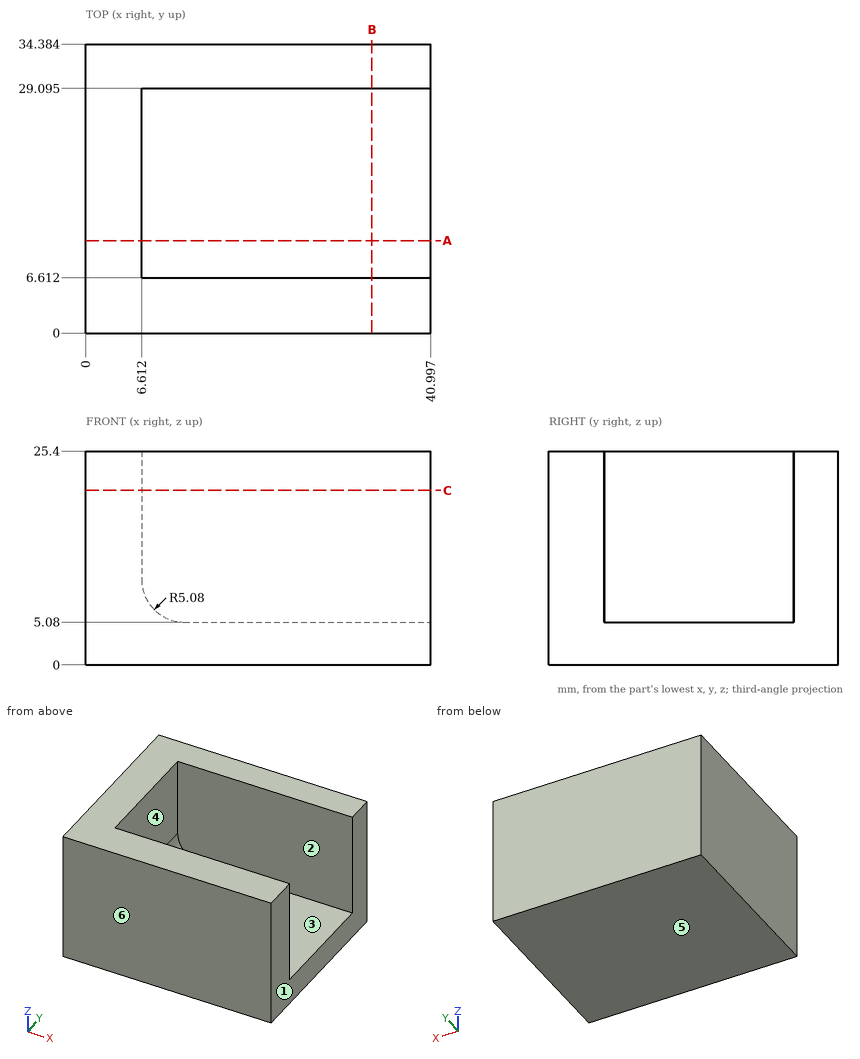
For this review, use the dimensioned drawing (mm, ordinates from the lowest corner) and the shaded views. A direction names the side the tool comes from. Round coordinates to 2 decimals unless told otherwise and drop trailing zeros. Write each loop counter-clockwise with the first axis right and the second up, starting at its lowest first coordinate (ties: lowest second). Pieces come first, ordered by that corner, then holes. Notation, with made-up numbers: M 59.25,44.25 L 75.25,44.25 A10 cw 75.25,49.25 Z; hole C 50,12 d1. An arc over 180 degrees is marked long. Answer as CSV lines item,"result". Start each with the question number.
Q1. Wall thickness on line 1 along Y through (x, z) = (17, 13.75) (1 decimal); line 2 along X through (y, z) = (28, 13.25); line 3 along Z through (x, y) = (36, 7): over which ranges is each line inside the solid? List them lowest first.
Q2. The part is to be moulded in two halves that separate along Y. For the marked faces 3, 4, 5 and 6, say which applies: +Y half, -Y half, draft (parallel to the pull), parting line (faces both ways), or undercut.
Q3. Consider section A-A, the plane y = 11. Give the boundary of the cut face in (x, z), then the cut area to 3 significant figures.
Q4. Clearance check with flat-ended pins moving along their axes: P1, Ø6.5, axis at x = 24, y = 13, coming from the +Z side; P2, Ø4.5, axis at y = 19, z = 15, coming from the +X side. State where each tip first meets the part, or that it passes through.
Q5. Consider section B-B, the plane x = 34. Give the boundary of the cut face in (y, z) (1 decimal).
Q6. Tool access review of the marked faces 1 and 2: name each direction out of +Z, -Z, +X, -X, +Y, -Y from which nothing blocks a thin tool from reaching the whole face with its end or side.
Q7. Consider section C-C, the plane z = 20.75. Give the boundary of the cut face in (x, y) (1 decimal).
Result set:
1,line 1,"y = 0 to 6.6, 29.1 to 34.4"
1,line 2,"x = 0 to 6.61"
1,line 3,"z = 0 to 5.08"
2,face 3,"undercut"
2,face 4,"undercut"
2,face 5,"draft"
2,face 6,"-Y half"
3,outline,"M 0,0 L 41,0 L 41,5.08 L 11.69,5.08 A5.08 cw 6.61,10.16 L 6.61,25.4 L 0,25.4 Z"
3,area,"348 mm²"
4,P1,"stops at z = 5.08"
4,P2,"stops at x = 6.61"
5,outline,"M 0,0 L 34.4,0 L 34.4,25.4 L 29.1,25.4 L 29.1,5.1 L 6.6,5.1 L 6.6,25.4 L 0,25.4 Z"
6,face 1,"+Z, -Z, +X, +Y, -Y"
6,face 2,"+Z, +X"
7,outline,"M 0,0 L 41,0 L 41,6.6 L 6.6,6.6 L 6.6,29.1 L 41,29.1 L 41,34.4 L 0,34.4 Z"
